from build123d import *

# Parameters (mm, degrees)
SKETCH1_W            = 27.25
SKETCH1_H            = 18.76
SKETCH1_W_2          = 23.25
SKETCH1_H_2          = 14.76
BOSS_EXTRUDE1_DEPTH  = 18
SKETCH3_W            = 23.25
SKETCH3_H            = 14.76
BOSS_EXTRUDE2_DEPTH  = 2
SKETCH7_W            = 2
SKETCH7_H            = 5
CUT_EXTRUDE1_DEPTH   = 2
SKETCH10_W           = 23.25
SKETCH10_H           = 14.76
SKETCH10_W_2         = 7
SKETCH10_H_2         = 18.76
BOSS_EXTRUDE3_DEPTH  = 2
SKETCH11_R           = 1.5
CUT_EXTRUDE3_DEPTH   = 2
SKETCH12_R           = 1.5
CUT_EXTRUDE4_DEPTH   = 2
FILLET11_R           = 1
SKETCH13_W           = 3
SKETCH13_H           = 18.76
CUT_EXTRUDE5_DEPTH   = 10
CUT_EXTRUDE6_REACH   = 42.094
SKETCH14_W           = 27.25
SKETCH14_H           = 8
SKETCH16_W           = 23.25
SKETCH16_H           = 2
BOSS_EXTRUDE5_DEPTH  = 7.6
SKETCH19_W           = 2
SKETCH19_H           = 0.99
CUT_EXTRUDE8_DEPTH   = 10
BOSS_EXTRUDE6_DEPTH  = 4
SKETCH21_R           = 1.25
CUT_EXTRUDE9_DEPTH   = 2
BOSS_EXTRUDE7_DEPTH  = 1
CUT_EXTRUDE11_START  = -12
CUT_EXTRUDE11_DEPTH  = 12
SKETCH26_W           = 28.086287418
SKETCH26_H           = 15.375704791
CUT_EXTRUDE13_DEPTH  = 4
SKETCH27_W           = 24.075870352
SKETCH27_H           = 3.872197668
CUT_EXTRUDE14_DEPTH  = 12
SKETCH28_W           = 5.439700639
SKETCH28_H           = 5.036759851
BOSS_EXTRUDE8_DEPTH  = 2
SKETCH29_R           = 1.25
CUT_EXTRUDE15_DEPTH  = 2
SKETCH30_W           = 2
SKETCH30_H           = 0.99
BOSS_EXTRUDE9_DEPTH  = 10
SKETCH32_W           = 3.854176667
SKETCH32_H           = 5.494251846
SKETCH32_W_2         = 4.510206738
SKETCH32_H_2         = 5.863268761
BOSS_EXTRUDE11_DEPTH = 2
BOSS_EXTRUDE13_START = -2
BOSS_EXTRUDE13_DEPTH = 2


with BuildPart() as part:
    # Sketch1 → Boss-Extrude1 (new body)
    with BuildSketch(Plane.XY):
        with Locations((11.625, -7.38)):
            Rectangle(SKETCH1_W, SKETCH1_H)
        with Locations((11.625, -7.38)):
            Rectangle(SKETCH1_W_2, SKETCH1_H_2, mode=Mode.SUBTRACT)
    extrude(amount=BOSS_EXTRUDE1_DEPTH)

    # Sketch3 → Boss-Extrude2 (add)
    with BuildSketch(Plane(origin=(0, 0, 0), x_dir=(-1, 0, 0), z_dir=(0, 0, -1))):
        with Locations((-11.625, -7.38)):
            Rectangle(SKETCH3_W, SKETCH3_H)
    extrude(amount=-BOSS_EXTRUDE2_DEPTH)

    # Sketch7 → Cut-Extrude1 (cut)
    with BuildSketch(Plane.ZY.offset(2)):
        with Locations((3, -6.5)):
            Rectangle(SKETCH7_W, SKETCH7_H)
    extrude(amount=-CUT_EXTRUDE1_DEPTH, mode=Mode.SUBTRACT)

    # Sketch10 → Boss-Extrude3 (add)
    # profile 1 of 3: a face of its own
    with BuildSketch(Plane.XY.offset(18)):
        Polygon((-2, -0.03961342), (-2, 2), (-9, 2), (-9, -16.76), (-2, -16.76), (-2, -13.03961342), align=None)
    # profile 2 of 3: a face of its own
    with BuildSketch(Plane.XY.offset(18)):
        Polygon((25.25, 2), (-2, 2), (-2, -0.03961342), (-2, -13.03961342), (-2, -16.76), (25.25, -16.76), align=None)
        with Locations((11.625, -7.38)):
            Rectangle(SKETCH10_W, SKETCH10_H, mode=Mode.SUBTRACT)
    # profile 3 of 3: a face of its own
    with BuildSketch(Plane.XY.offset(18)):
        with Locations((28.75, -7.38)):
            Rectangle(SKETCH10_W_2, SKETCH10_H_2)
    extrude(amount=BOSS_EXTRUDE3_DEPTH)

    # Sketch11 → Cut-Extrude3 (cut)
    with BuildSketch(Plane(origin=(0, 0, 18), x_dir=(-1, 0, 0), z_dir=(0, 0, -1))):
        with Locations((3.5, -8.26)):
            Circle(SKETCH11_R)
    extrude(amount=-CUT_EXTRUDE3_DEPTH, mode=Mode.SUBTRACT)

    # Sketch12 → Cut-Extrude4 (cut)
    with BuildSketch(Plane(origin=(0, 0, 18), x_dir=(-1, 0, 0), z_dir=(0, 0, -1))):
        with Locations((-26.95, -8.26)):
            Circle(SKETCH12_R)
    extrude(amount=-CUT_EXTRUDE4_DEPTH, mode=Mode.SUBTRACT)

    # Fillet11
    fillet11_edges = [part.edges().sort_by_distance(p)[0] for p in [
        (0, -9, 3),
        (0, -4, 3),
        (0, -6.5, 4),
        (-2, -6.5, 4),
        (-2, -4, 3),
        (-2, -9, 3),
    ]]
    fillet(fillet11_edges, radius=FILLET11_R - 0.0001)  # a hair under: the kernel refuses the full size

    # Sketch13 → Cut-Extrude5 (cut)
    with BuildSketch(Plane(origin=(0, 0, 18), x_dir=(-1, 0, 0), z_dir=(0, 0, -1))):
        with Locations((-30.75, -7.38)):
            Rectangle(SKETCH13_W, SKETCH13_H)
        with Locations((7.5, -7.38)):
            Rectangle(SKETCH13_W, SKETCH13_H)
    extrude(amount=-CUT_EXTRUDE5_DEPTH, mode=Mode.SUBTRACT)

    # Cut-Extrude6: up to this face of the body (flat: up to its plane)
    cut_extrude6_end = Plane(part.part.faces().sort_by_distance((11.625, -16.76, 10.256684492))[0])
    # Sketch14 → Cut-Extrude6 (cut, up to the picked face)
    with BuildSketch(Plane(origin=(0, 2, 0), x_dir=(1, 0, 0), z_dir=(0, 1, 0)), mode=Mode.PRIVATE) as cut_extrude6_sk1:
        with Locations((11.625, -4)):
            Rectangle(SKETCH14_W, SKETCH14_H)
    cut_extrude6_tool1 = split(extrude(cut_extrude6_sk1.sketch, amount=-CUT_EXTRUDE6_REACH, mode=Mode.PRIVATE), bisect_by=cut_extrude6_end, keep=Keep.BOTH, mode=Mode.PRIVATE)
    add(cut_extrude6_tool1.solids().sort_by(Axis((11.625, 2, 4), (0, -1, 0)))[0], mode=Mode.SUBTRACT)

    # Sketch16 → Boss-Extrude5 (add)
    with BuildSketch(Plane.XY.offset(20)):
        with Locations((11.625, -15.76)):
            Rectangle(SKETCH16_W, SKETCH16_H)
    extrude(amount=BOSS_EXTRUDE5_DEPTH)

    # Sketch19 → Cut-Extrude8 (cut)
    with BuildSketch(Plane(origin=(0, 0, 8), x_dir=(-1, 0, 0), z_dir=(0, 0, -1))):
        with Locations((1, -7.255)):
            Rectangle(SKETCH19_W, SKETCH19_H)
        with Locations((-24.25, -7.255)):
            Rectangle(SKETCH19_W, SKETCH19_H)
    extrude(amount=-CUT_EXTRUDE8_DEPTH, mode=Mode.SUBTRACT)

    # Sketch20 → Boss-Extrude6 (add)
    with BuildSketch(Plane.XZ.offset(16.76)):
        with BuildLine():
            ThreePointArc((1.734487906, 14.866457564), (-0.15, 17.000000025), (1.734487955, 19.133542442))
            Line((1.734487955, 19.133542442), (4.661486136, 19.497797339))
            ThreePointArc((4.661486136, 19.497797339), (3.240091566, 20.432881138), (1.549246975, 20.622060423))
            ThreePointArc((1.549246975, 20.622060423), (0.742054746, 20.4263791), (0, 20.053276928))
            Line((0, 20.053276928), (0, 20))
            Line((0, 20), (-0.079062289, 20))
            ThreePointArc((-0.079062289, 20), (-1.544419903, 16.128456799), (1.549246968, 13.377939578))
            ThreePointArc((1.549246968, 13.377939578), (3.240091563, 13.567118861), (4.661486136, 14.502202661))
            Line((4.661486136, 14.502202661), (1.734487906, 14.866457564))
        make_face()
        with BuildLine():
            ThreePointArc((1.549246975, 20.622060423), (3.240091566, 20.432881138), (4.661486136, 19.497797339))
            Line((4.661486136, 19.497797339), (14.257253364, 20.691957699))
            ThreePointArc((14.257253364, 20.691957699), (15.89224684, 22.015782374), (17.896084422, 22.656368345))
            Line((17.896084422, 22.656368345), (1.549246975, 20.622060423))
        make_face()
        with BuildLine():
            ThreePointArc((17.896084422, 22.656368345), (15.89224684, 22.015782374), (14.257253364, 20.691957699))
            Line((14.257253364, 20.691957699), (18.081325153, 21.167850334))
            ThreePointArc((18.081325153, 21.167850334), (21.380428532, 20.14789091), (22.8, 17))
            ThreePointArc((22.8, 17), (21.380428595, 13.852109147), (18.081325321, 12.832149645))
            Line((18.081325321, 12.832149645), (14.257253364, 13.308042301))
            ThreePointArc((14.257253364, 13.308042301), (15.89224684, 11.984217626), (17.896084422, 11.343631655))
            ThreePointArc((17.896084422, 11.343631655), (22.37343883, 12.727862432), (24.3, 17))
            ThreePointArc((24.3, 17), (24.082512903, 18.559503854), (23.446648326, 20))
            Line((23.446648326, 20), (23.25, 20))
            Line((23.25, 20), (23.25, 20.296589146))
            ThreePointArc((23.25, 20.296589146), (20.898920406, 22.215837897), (17.896084422, 22.656368345))
        make_face()
        with BuildLine():
            Line((14.257253364, 13.308042301), (4.661486136, 14.502202661))
            ThreePointArc((4.661486136, 14.502202661), (3.240091563, 13.567118861), (1.549246968, 13.377939578))
            Line((1.549246968, 13.377939578), (17.896084422, 11.343631655))
            ThreePointArc((17.896084422, 11.343631655), (15.89224684, 11.984217626), (14.257253364, 13.308042301))
        make_face()
    extrude(amount=BOSS_EXTRUDE6_DEPTH)

    # Sketch21 → Cut-Extrude9 (cut)
    with BuildSketch(Plane.XZ.offset(16.76)):
        with Locations((18.6, 17)):
            Circle(SKETCH21_R)
    extrude(amount=-CUT_EXTRUDE9_DEPTH, mode=Mode.SUBTRACT)

    # Sketch23 → Boss-Extrude7 (add)
    with BuildSketch(Plane.XZ.offset(16.76)):
        Polygon((11.1, 21.100651295), (0.406174607, 19.998863224), (-0.954500861, 17.320033397), (0.387681288, 14.425953139), (11.1, 12.86779769), align=None)
    extrude(amount=BOSS_EXTRUDE7_DEPTH)

    # Sketch24 → Cut-Extrude11 (cut)
    with BuildSketch(Plane.XZ.offset(16.76).offset(CUT_EXTRUDE11_START)):
        with BuildLine():
            ThreePointArc((0, 20.053276928), (0.742054739, 20.426379098), (1.549246961, 20.622060422))
            Line((1.549246961, 20.622060422), (17.896084422, 22.656368345))
            ThreePointArc((17.896084422, 22.656368345), (20.898920406, 22.215837897), (23.25, 20.296589146))
            Line((23.25, 20.296589146), (23.25, 27.6))
            Line((23.25, 27.6), (0, 27.6))
            Line((0, 27.6), (0, 20.053276928))
        make_face()
    extrude(amount=CUT_EXTRUDE11_DEPTH, mode=Mode.SUBTRACT)

    # Sketch26 → Cut-Extrude13 (cut)
    with BuildSketch(Plane.XZ.offset(20.76)):
        with Locations((10.743459592, 18.384139078)):
            Rectangle(SKETCH26_W, SKETCH26_H)
    extrude(amount=-CUT_EXTRUDE13_DEPTH, mode=Mode.SUBTRACT)

    # Sketch27 → Cut-Extrude14 (cut)
    with BuildSketch(Plane(origin=(0, -16.76, 0), x_dir=(-1, 0, 0), z_dir=(0, -1, 0))):
        with Locations((-12.037935176, -21.936098834)):
            Rectangle(SKETCH27_W, SKETCH27_H)
    extrude(amount=-CUT_EXTRUDE14_DEPTH, mode=Mode.SUBTRACT)

    # Sketch28 → Boss-Extrude8 (add)
    with BuildSketch(Plane.XZ.offset(16.76)):
        with Locations((19.018963462, 16.417644729)):
            Rectangle(SKETCH28_W, SKETCH28_H)
    extrude(amount=-BOSS_EXTRUDE8_DEPTH)

    # Sketch29 → Cut-Extrude15 (cut)
    with BuildSketch(Plane(origin=(0, 2, 0), x_dir=(1, 0, 0), z_dir=(0, 1, 0))):
        with Locations(Location((2, -11, 0), (0, 0, 270))):
            Circle(SKETCH29_R)
        with Locations(Location((21.25, -11, 0), (0, 0, 270))):
            Circle(SKETCH29_R)
        with Locations(Location((2, -17, 0), (0, 0, 270))):
            Circle(SKETCH29_R)
        with Locations(Location((21.25, -17, 0), (0, 0, 270))):
            Circle(SKETCH29_R)
    extrude(amount=-CUT_EXTRUDE15_DEPTH, mode=Mode.SUBTRACT)

    # Sketch30 → Boss-Extrude9 (add)
    with BuildSketch(Plane(origin=(0, 0, 18), x_dir=(-1, 0, 0), z_dir=(0, 0, -1))):
        with Locations((-24.25, -7.255)):
            Rectangle(SKETCH30_W, SKETCH30_H)
        with Locations((1, -7.255)):
            Rectangle(SKETCH30_W, SKETCH30_H)
    extrude(amount=BOSS_EXTRUDE9_DEPTH)

    # Sketch32 → Boss-Extrude11 (add)
    with BuildSketch(Plane.XY.offset(20)):
        with Locations((-3.545695394, -6.231493422)):
            Rectangle(SKETCH32_W, SKETCH32_H)
        with Locations((26.590685996, -6.046984965)):
            Rectangle(SKETCH32_W_2, SKETCH32_H_2)
    extrude(amount=-BOSS_EXTRUDE11_DEPTH)

    # Sketch33 → Boss-Extrude13 (add)
    with BuildSketch(Plane.XY.offset(20).offset(BOSS_EXTRUDE13_START)):
        with BuildLine():
            Line((-2.183342779, -8.978619345), (-2.848663443, -8.978619345))
            Line((-2.848663443, -8.978619345), (-2.848663443, -9.611207123))
            ThreePointArc((-2.848663443, -9.611207123), (-2.466418023, -9.347064073), (-2.183342779, -8.978619345))
        make_face()
        with BuildLine():
            Line((-2.848663443, -9.611207123), (-2.848663443, -8.978619345))
            Line((-2.848663443, -8.978619345), (-4.816657221, -8.978619345))
            ThreePointArc((-4.816657221, -8.978619345), (-3.959025839, -9.688038963), (-2.848663443, -9.611207123))
        make_face()
        with BuildLine():
            ThreePointArc((28.266657221, -8.978619345), (26.95, -9.76), (25.633342779, -8.978619345))
            Line((25.633342779, -8.978619345), (28.266657221, -8.978619345))
        make_face()
    extrude(amount=BOSS_EXTRUDE13_DEPTH)


solid = part.part
Design review of the part built by this model. Coordinates are the model's own, in mm. A direction names the side the tool comes from. Coordinates: 2 decimals unless noted, no trailing zeros. Write each loop counter-clockwise with the first axis right and the second up, starting at its lowest first coordinate (ties: lowest second). Pieces come first, ordered by that corner, then holes. Notation, with made-up numbers: (63.5, -15.75) - (118.5, -15.75) arc R25 cw to (118.5, 12.25) - close; hole circle Ø7 at (88, 39.5). An arc over 180 degrees is marked (long way). One line per item, written item: value.
1) Mouldability with a two-part tool opening along X and no side actions: class faces 5 (the face through (-2, -8, 13)), 6 (the face through (25.25, -8, 13)), 7 (the face through (12, -16, 8)), 8 (the face through (20, 1, 17)) as +X half, -X half, draft (parallel to the pull), parting line (faces both ways), or undercut.
Answer sheet:
face 5: -X half
face 6: +X half
face 7: draft
face 8: undercut
2) Add section D-D (z = 19). State the section outline as (x, y) points.
Answer sheet:
outline: (-6, -16.76) - (29.25, -16.76) - (29.25, 2) - (-6, 2) - close; hole (0, -14.76) - (23.25, -14.76) - (23.25, 0) - (0, 0) - close
3) Add section B-B (y = -5). State the section outline as (x, z) points, plus the area to 3 significant figures.
Answer sheet:
outline: (-6, 18) - (-2, 18) - (-2, 8) - (0, 8) - (0, 20) - (-6, 20) - close; (23.25, 8) - (25.25, 8) - (25.25, 18) - (29.25, 18) - (29.25, 20) - (23.25, 20) - close
area: 64.0 mm2
4) For faces 1 (the face through (-4, -7, 18)), 2 (the face through (2.05, 1.01, 9.75)), 3 (the face through (27, -7, 18)), 4 (the face through (11, 0, 14)), list the 3-axis set-ups (+Z, -Z, +X, -X, +Y, -Y) from which the entire face can be reached by the end or side of a thin tool; tool diameter is ignored.
Answer sheet:
face 1: -Z, -X, +Y, -Y
face 2: +Y
face 3: -Z, +X, +Y, -Y
face 4: +Z, -Z
5) Add section C-C (x = 16). State the section outline as (y, z) points.
Answer sheet:
outline: (-16.76, 8) - (-14.76, 8) - (-14.76, 20) - (-16.76, 20) - close; (0, 8) - (2, 8) - (2, 20) - (0, 20) - close
6) Insertion check: pin 1 (2 mm diameter, centred on x = -4.5, y = -6, fed in from -Z); pin 2 (3 mm diameter, centred on y = -4.5, z = 13.5, fed in from -X); pin 3 (1.5 mm diameter, centred on y = -10, z = 15.5, fed in from +X). Each pin has a flat end and moves straight along its axis. Give the tip position at first contact, or say it passes through.
Answer sheet:
pin 1: stops at z = 18
pin 2: stops at x = -2
pin 3: stops at x = 25.25
7) To check wall thickness, follow probe 1 along X at (y, z) = (0.5, 17); probe 2 along Y at (x, z) = (12, 10.75); probe 3 along X at (y, z) = (-12, 11.5). State the ranges of each line that lie inside material, in increasing order.
Answer sheet:
probe 1: x = -2 to 0.75, 3.25 to 20, 22.5 to 25.25
probe 2: y = -16.76 to -14.76, 0 to 2
probe 3: x = -2 to 0, 23.25 to 25.25
8) Add section A-A (z = 17). State the section outline as (x, y) points, plus the area to 3 significant figures.
Answer sheet:
outline: (-2, -16.76) - (25.25, -16.76) - (25.25, 2) - (22.5, 2) - (22.5, 0) - (23.25, 0) - (23.25, -14.76) - (0, -14.76) - (0, 0) - (0.75, 0) - (0.75, 2) - (-2, 2) - close; (3.25, 0) - (20, 0) - (20, 2) - (3.25, 2) - close
area: 158 mm2
